from build123d import *

# Parameters (mm, degrees)
SKETCH1_W             = 26
SKETCH1_H             = 70
BOSS_EXTRUDE1_DEPTH   = 40
FILLET1_R             = 3
CUT_EXTRUDE1_REACH    = 56.717
M8_TAPPED_HOLE1_D     = 6.8
M8_TAPPED_HOLE1_DEPTH = 22.25
M8_TAPPED_HOLE1_TIP   = 2.042926105


with BuildPart() as part:
    # Sketch1 → Boss-Extrude1 (new body)
    with BuildSketch(Plane(origin=(0, 0, 0), x_dir=(1, 0, 0), z_dir=(0, 1, 0))):
        Rectangle(SKETCH1_W, SKETCH1_H)
    extrude(amount=-BOSS_EXTRUDE1_DEPTH)

    # Fillet1
    fillet1_edges = [part.edges().sort_by_distance(p)[0] for p in [
        (13, -20, 35),
        (-13, -20, 35),
        (-13, -20, -35),
        (13, -20, -35),
    ]]
    fillet(fillet1_edges, radius=FILLET1_R)

    # Sketch9 → Cut-Extrude1 (cut, up to next)
    with BuildSketch(Plane(origin=(0, 0, 0), x_dir=(1, 0, 0), z_dir=(0, 1, 0)), mode=Mode.PRIVATE) as cut_extrude1_sk1:
        with BuildLine():
            Line((3.08, 9), (3.08, -9))
            ThreePointArc((3.08, -9), (2.508858223, -10.378858223), (1.13, -10.95))
            Line((1.13, -10.95), (-5, -10.95))
            ThreePointArc((-5, -10.95), (-7.156675683, -11.843324317), (-8.05, -14))
            Line((-8.05, -14), (-8.05, -16.05))
            Line((-8.05, -16.05), (5.13, -16.05))
            ThreePointArc((5.13, -16.05), (7.286675683, -15.156675683), (8.18, -13))
            Line((8.18, -13), (8.18, 13))
            ThreePointArc((8.18, 13), (7.286675683, 15.156675683), (5.13, 16.05))
            Line((5.13, 16.05), (-8.05, 16.05))
            Line((-8.05, 16.05), (-8.05, 14))
            ThreePointArc((-8.05, 14), (-7.156675683, 11.843324317), (-5, 10.95))
            Line((-5, 10.95), (1.13, 10.95))
            ThreePointArc((1.13, 10.95), (2.508858223, 10.378858223), (3.08, 9))
        make_face()
    cut_extrude1_tool1 = extrude(cut_extrude1_sk1.sketch, amount=-CUT_EXTRUDE1_REACH, mode=Mode.PRIVATE) & part.part
    add(cut_extrude1_tool1.solids().sort_by_distance((3.439697, 0, 0))[0], mode=Mode.SUBTRACT)

    # Cut-Sweep1: sweep along a path in Sketch12
    with BuildLine(Plane(origin=(0, 0, 0), x_dir=(1, 0, 0), z_dir=(0, 1, 0))) as cut_sweep1_path:
        Line((-8.05, -14), (-8.05, -16.05))
        Line((-8.05, -16.05), (5.13, -16.05))
        ThreePointArc((5.13, -16.05), (7.286675683, -15.156675683), (8.18, -13))
        Line((8.18, -13), (8.18, 13))
        ThreePointArc((8.18, 13), (7.286675683, 15.156675683), (5.13, 16.05))
        Line((5.13, 16.05), (-8.05, 16.05))
        Line((-8.05, 16.05), (-8.05, 14))
        ThreePointArc((-8.05, 14), (-7.156675683, 11.843324317), (-5, 10.95))
        Line((-5, 10.95), (1.13, 10.95))
        ThreePointArc((1.13, 10.95), (2.508858223, 10.378858223), (3.08, 9))
        Line((3.08, 9), (3.08, -9))
        ThreePointArc((3.08, -9), (2.508858223, -10.378858223), (1.13, -10.95))
        Line((1.13, -10.95), (-5, -10.95))
        ThreePointArc((-5, -10.95), (-7.156675683, -11.843324317), (-8.05, -14))
    # Sketch11 → Cut-Sweep1 (sweep, cut)
    with BuildSketch(Plane.XY):
        Polygon((8.18, -3.2), (8.822346389, -40), (8.18, -40), align=None)
    sweep(path=cut_sweep1_path.line, transition=Transition.RIGHT, mode=Mode.SUBTRACT)

    # M8 Tapped Hole1
    with Locations(Plane(origin=(0, -40, 0), x_dir=(-1, 0, 0), z_dir=(0, -1, 0))):
        with Locations((0, -25.846173195), (0, 25.846173195)):
            Hole(M8_TAPPED_HOLE1_D / 2, depth=M8_TAPPED_HOLE1_DEPTH)
            with Locations((0, 0, -(M8_TAPPED_HOLE1_DEPTH + M8_TAPPED_HOLE1_TIP / 2))):  # 118° drill point
                Cone(0, M8_TAPPED_HOLE1_D / 2, M8_TAPPED_HOLE1_TIP, mode=Mode.SUBTRACT)


solid = part.part
The model under review builds one solid part; all positions refer to its coordinate system, in mm. A direction names the side the tool comes from. Round coordinates to 2 decimals unless told otherwise and drop trailing zeros. Loops run counter-clockwise (first coordinate to the right, second up) from the corner with the lowest first, then second, coordinate; pieces in that order, holes last. Notation, with made-up numbers: M 72.25,-22.75 L 88.25,-22.75 A27 ccw 88.25,6.25 Z; hole C -31.5,-10 d2. An arc over 180 degrees is marked long. Answer as CSV lines item,"result". Start each with the question number.
Item 1: Mouldability with a two-part tool opening along X and no side actions: class faces 1 (the face through (-12.14, -20.28, -34.1)), 2 (the face through (-8.05, -2, 15)), 3 (the face through (0, -20, 35)) as released by +X, released by -X, zero draft, split by the parting line, or undercut.
Item 2: Consider section D-D (y = -22). Write out the cut boundary in (x, z), then the cut area to 3 significant figures.
Item 3: For faces 4 (the face through (12.1, -20.28, 34.14)), 5 (the face through (-8.05, -2, -15)), 6 (the face through (2.3, -21.34, 10.14)), list the 3-axis set-ups (+Z, -Z, +X, -X, +Y, -Y) from which the entire face can be reached by the end or side of a thin tool; tool diameter is ignored.
Item 4: Wall thickness on line 1 (Z direction, x = 0, y = -23.5); line 2 (Z direction, x = 0, y = -32.5); line 3 (X direction, y = -4, z = 1): over which ranges is each line inside the solid? List them lowest first. Write a range as [from, to].
Item 5: Consider section C-C (x = -2.25). State how many separate pieces and enclosed holes the cut face has, then the cut area to 3 significant figures.
Item 6: Consider section A-A (z = 0). Write out the cut boundary in (x, y).
Item 7: Consider section B-B (y = -28.5). Write out the cut boundary in (x, z), then the cut area to 3 significant figures.
Item 8: Insertion check: P1, Ø6, axis at x = 0, z = -25.85, coming from the -Y side. The pin has a flat end and moves straight along its axis. Give the tip position at first contact, or say it passes through.
Answer:
1,face 1,"released by -X"
1,face 2,"undercut"
1,face 3,"zero draft"
2,outline,"M -13,-32 A3 ccw -10,-35 L 10,-35 A3 ccw 13,-32 L 13,32 A3 ccw 10,35 L -10,35 A3 ccw -13,32 Z; hole M -8.38,-16.38 L 5.13,-16.38 A3.38 ccw 8.51,-13 L 8.51,13 A3.38 ccw 5.13,16.38 L -8.38,16.38 L -8.38,14 A3.38 ccw -5,10.62 L 1.13,10.62 A1.62 cw 2.75,9 L 2.75,-9 A1.62 cw 1.13,-10.62 L -5,-10.62 A3.38 ccw -8.38,-14 Z; hole C 0,-25.85 d6.8; hole C 0,25.85 d6.8"
2,area,"1,430 mm^2"
3,face 4,"+Z, +X, +Y, -Y"
3,face 5,"+Y, -Y"
3,face 6,"-Y"
4,line 1,"z = [-35, -29.25], [-22.45, -16.4], [-10.6, 10.6], [16.4, 22.45], [29.25, 35]"
4,line 2,"z = [-35, -29.25], [-22.45, -16.56], [-10.44, 10.44], [16.56, 22.45], [29.25, 35]"
4,line 3,"x = [-13, 3.07], [8.19, 13]"
5,separate pieces,"3"
5,enclosed holes,"0"
5,area,"2,110 mm^2"
6,outline,"M -13,-40 L 2.44,-40 L 3.08,-3.2 L 3.08,0 L -13,0 Z; M 8.18,-3.2 L 8.82,-40 L 13,-40 L 13,0 L 8.18,0 Z"
7,outline,"M -13,-32 A3 ccw -10,-35 L 10,-35 A3 ccw 13,-32 L 13,32 A3 ccw 10,35 L -10,35 A3 ccw -13,32 Z; hole M -8.49,-16.49 L 5.13,-16.49 A3.49 ccw 8.62,-13 L 8.62,13 A3.49 ccw 5.13,16.49 L -8.49,16.49 L -8.49,14 A3.49 ccw -5,10.51 L 1.13,10.51 A1.51 cw 2.64,9 L 2.64,-9 A1.51 cw 1.13,-10.51 L -5,-10.51 A3.49 ccw -8.49,-14 Z; hole C 0,-25.85 d6.8; hole C 0,25.85 d6.8"
7,area,"1,420 mm^2"
8,P1,"stops at y = -17.51"
